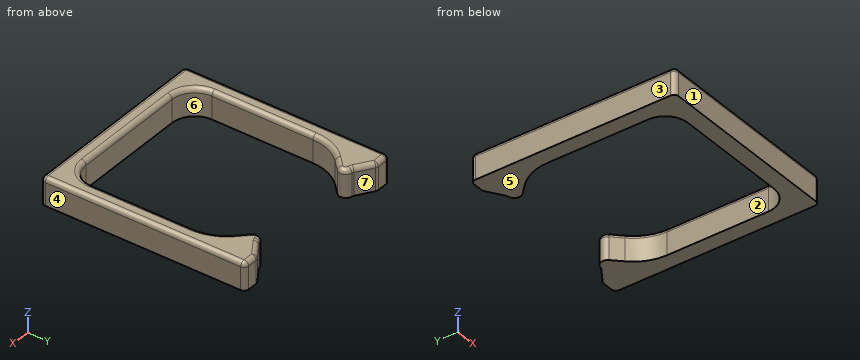
```python
from build123d import *

# Parameters (mm, degrees)
BOSS_EXTRUDE1_DEPTH = 6
FILLET2_R           = 1


with BuildPart() as part:
    # Sketch1 → Boss-Extrude1 (new body)
    with BuildSketch(Plane.XY):
        with BuildLine():
            ThreePointArc((-157.718887647, -39.971100876), (-157.425994428, -40.678207657), (-156.718887647, -40.971100876))
            Line((-156.718887647, -40.971100876), (-154.209280647, -40.971100876))
            Line((-154.209280647, -40.971100876), (-118.966369371, -40.971100876))
            Line((-118.966369371, -40.971100876), (-116.875365395, -40.971100876))
            Line((-116.875365395, -40.971100876), (-116.456762371, -40.971100876))
            ThreePointArc((-116.456762371, -40.971100876), (-115.749655589, -40.678207657), (-115.456762371, -39.971100876))
            Line((-115.456762371, -39.971100876), (-115.456762371, 3.028899124))
            ThreePointArc((-115.456762371, 3.028899124), (-115.749655589, 3.736005905), (-116.456762371, 4.028899124))
            Line((-116.456762371, 4.028899124), (-118.668700725, 4.028899124))
            ThreePointArc((-118.668700725, 4.028899124), (-118.953997988, 3.987338205), (-119.215580818, 3.866110067))
            Line((-119.215580818, 3.866110067), (-122.622400092, 1.640719134))
            ThreePointArc((-122.622400092, 1.640719134), (-122.820936659, 1.540563133), (-123.036698115, 1.486758046))
            ThreePointArc((-123.036698115, 1.486758046), (-124.259059599, 0.479679308), (-123.896981272, -1.062161951))
            Line((-123.896981272, -1.062161951), (-121.905327613, -3.048179664))
            ThreePointArc((-121.905327613, -3.048179664), (-119.730287475, -6.295880771), (-118.966369371, -10.129259334))
            Line((-118.966369371, -10.129259334), (-118.966369371, -32.384364229))
            ThreePointArc((-118.966369371, -32.384364229), (-120.430835465, -35.919898135), (-123.966369371, -37.384364229))
            Line((-123.966369371, -37.384364229), (-149.209280647, -37.384364229))
            ThreePointArc((-149.209280647, -37.384364229), (-152.744814552, -35.919898135), (-154.209280647, -32.384364229))
            Line((-154.209280647, -32.384364229), (-154.209280647, -10.129259334))
            ThreePointArc((-154.209280647, -10.129259334), (-153.445362542, -6.295880771), (-151.270322404, -3.048179664))
            Line((-151.270322404, -3.048179664), (-149.278668745, -1.062161951))
            ThreePointArc((-149.278668745, -1.062161951), (-148.916590418, 0.479679308), (-150.138951903, 1.486758046))
            ThreePointArc((-150.138951903, 1.486758046), (-150.354713358, 1.540563133), (-150.553249925, 1.640719134))
            Line((-150.553249925, 1.640719134), (-153.960069199, 3.866110067))
            ThreePointArc((-153.960069199, 3.866110067), (-154.221652029, 3.987338205), (-154.506949292, 4.028899124))
            Line((-154.506949292, 4.028899124), (-156.718887647, 4.028899124))
            ThreePointArc((-156.718887647, 4.028899124), (-157.425994428, 3.736005905), (-157.718887647, 3.028899124))
            Line((-157.718887647, 3.028899124), (-157.718887647, -39.971100876))
        make_face()
    extrude(amount=BOSS_EXTRUDE1_DEPTH)

    # Fillet2
    fillet2_edges = [part.edges().sort_by_distance(p)[0] for p in [
        (-122.820936659, 1.540563133, 6),
        (-124.259059599, 0.479679308, 6),
        (-154.209280647, -21.256811782, 6),
        (-122.901154442, -2.055170807, 6),
        (-119.730287475, -6.295880771, 6),
        (-118.966369371, -21.256811782, 6),
        (-120.430835465, -35.919898135, 6),
        (-136.587825009, -37.384364229, 6),
        (-153.445362542, -6.295880771, 6),
        (-150.274495575, -2.055170807, 6),
        (-148.916590418, 0.479679308, 6),
        (-150.354713358, 1.540563133, 6),
        (-152.256659562, 2.7534146, 6),
        (-154.221652029, 3.987338205, 6),
        (-155.612918469, 4.028899124, 6),
        (-157.425994428, 3.736005905, 6),
        (-157.718887647, -18.471100876, 6),
        (-152.744814552, -35.919898135, 6),
        (-157.425994428, -40.678207657, 6),
        (-136.587825009, -40.971100876, 6),
        (-115.749655589, -40.678207657, 6),
        (-115.456762371, -18.471100876, 6),
        (-115.749655589, 3.736005905, 6),
        (-117.562731548, 4.028899124, 6),
        (-118.953997988, 3.987338205, 6),
        (-120.918990455, 2.7534146, 6),
    ]]
    fillet(fillet2_edges, radius=FILLET2_R)


solid = part.part
```
Verification items for the finished model (mm, model axes). Face numbers are marked on the shaded views. A direction names the side the tool comes from. Give positions to 0.01 mm unless a question says otherwise; leave off trailing zeros. Loops run counter-clockwise (first coordinate to the right, second up) from the corner with the lowest first, then second, coordinate; pieces in that order, holes last. Notation, with made-up numbers: M -33,-25 L -25,-25 A17 ccw -25,2 Z; hole C 71.25,65.5 d1. An arc over 180 degrees is marked long. One line per question, with ' | ' between items.
Item 1: Tool access check on the marked faces 5, 6 and 7. Record the directions out of +Z, -Z, +X, -X, +Y, -Y that give a thin tool (end or side, any length) a straight path to the whole face; none if there is none.
Completed:
face 5: -Z, +X, -X, +Y, -Y | face 6: +Z, -Z | face 7: +Z, -Z, +Y
Item 2: Thickness scan on line 1 (X direction, y = -19.5, z = 2.5); line 2 (X direction, y = -9, z = 4.25); line 3 (Y direction, x = -129, z = 5). Record the ranges inside material, lowest first. Write a range as [from, to].
Completed:
line 1: x = [-157.72, -154.21], [-118.97, -115.46] | line 2: x = [-157.72, -154.15], [-119.03, -115.46] | line 3: y = [-40.97, -37.38]
Item 3: Draft check along X on the marked faces 1, 2, 3 and 4. Enter one of: +X half, -X half, draft (parallel to the pull), parting line (faces both ways), or undercut.
Completed:
face 1: draft | face 2: undercut | face 3: -X half | face 4: +X half
Item 4: Depth check by flat-ended pin: P1, Ø4, axis at x = -150.5, y = -34, coming from the -Z side; P2, Ø2.5, axis at x = -137.5, z = 3.5, coming from the +Y side. Enter the tip coordinate at first touch or a pass-through.
Completed:
P1: passes through | P2: stops at y = -37.38
Item 5: Section check B-B, the plane z = 2.75. Record the cut outline in (x, y).
Completed:
outline: M -157.72,-39.97 A1 ccw -156.72,-40.97 L -116.46,-40.97 A1 ccw -115.46,-39.97 L -115.46,3.03 A1 ccw -116.46,4.03 L -118.67,4.03 A1 ccw -119.22,3.87 L -122.62,1.64 A1 cw -123.04,1.49 A1.5 ccw -123.9,-1.06 L -121.91,-3.05 A10 cw -118.97,-10.13 L -118.97,-32.38 A5 cw -123.97,-37.38 L -149.21,-37.38 A5 cw -154.21,-32.38 L -154.21,-10.13 A10 cw -151.27,-3.05 L -149.28,-1.06 A1.5 ccw -150.14,1.49 A1 cw -150.55,1.64 L -153.96,3.87 A1 ccw -154.51,4.03 L -156.72,4.03 A1 ccw -157.72,3.03 Z
Item 6: Section check C-C, the plane x = -146.5. Record the cut outline in (y, z).
Completed:
outline: M -40.97,0 L -37.38,0 L -37.38,5 A1 ccw -38.38,6 L -39.97,6 A1 ccw -40.97,5 Z
Item 7: Section check A-A, the plane y = -15.5. Record the cut outline in (x, z).
Completed:
outline: M -157.72,0 L -154.21,0 L -154.21,5 A1 ccw -155.21,6 L -156.72,6 A1 ccw -157.72,5 Z; M -118.97,0 L -115.46,0 L -115.46,5 A1 ccw -116.46,6 L -117.97,6 A1 ccw -118.97,5 Z
